from build123d import *

# Parameters (mm, degrees)
F0_W      = 125
F0_H      = 40
F1_DEPTH  = 3
F2_W      = 125
F2_H      = 3
F3_DEPTH  = 85
F4_W      = 125
F4_H      = 40
F5_DEPTH  = 3
F6_R      = 35
F7_DEPTH  = 25
F10_R     = 24
F8_R      = 38
F12_R     = 12.5
F13_DEPTH = 70.6
F16_R     = 18
F14_R     = 35
F18_W     = 70
F18_H     = 3
F19_DEPTH = 85
F20_W     = 60
F20_H     = 60
F21_DEPTH = 15.5
F22_W     = 3
F22_H     = 85
F23_DEPTH = 26
F24_R     = 5
F25_DEPTH = 9.5
F26_R     = 10
F27_DEPTH = 25


with BuildPart() as f1:
    # F0 (on Front) → F1 (new body)
    with BuildSketch(Plane.XZ):
        Rectangle(F0_W, F0_H)
        with BuildLine():
            ThreePointArc((62.5, -20), (82.5, 0), (62.5, 20))
            Line((62.5, 20), (62.5, -20))
        make_face()
        with BuildLine():
            Line((-62.5, -20), (-62.5, 20))
            ThreePointArc((-62.5, 20), (-82.5, 0), (-62.5, -20))
        make_face()
    extrude(amount=F1_DEPTH)

    # F2 (on face) → F3 (join)
    with BuildSketch(Plane.XZ.offset(3)):
        with Locations((0, 18.5)):
            Rectangle(F2_W, F2_H)
        with BuildLine():
            Line((-62.5, 17), (-62.5, 20))
            ThreePointArc((-62.5, 20), (-76.6421356237, 14.1421356237), (-82.5, 0))
            Line((-82.5, 0), (-79.5, 0))
            ThreePointArc((-79.5, 0), (-74.5208152802, 12.0208152802), (-62.5, 17))
        make_face()
        with BuildLine():
            ThreePointArc((82.5, 0), (76.6421356237, 14.1421356237), (62.5, 20))
            Line((62.5, 20), (62.5, 17))
            ThreePointArc((62.5, 17), (74.5208152802, 12.0208152802), (79.5, 0))
            Line((79.5, 0), (82.5, 0))
        make_face()
    extrude(amount=F3_DEPTH)

    # F4 (on face) → F5 (join)
    with BuildSketch(Plane.XZ.offset(88)):
        Rectangle(F4_W, F4_H)
        with BuildLine():
            Line((-62.5, -20), (-62.5, 20))
            ThreePointArc((-62.5, 20), (-82.5, 0), (-62.5, -20))
        make_face()
        with BuildLine():
            ThreePointArc((62.5, -20), (82.5, 0), (62.5, 20))
            Line((62.5, 20), (62.5, -20))
        make_face()
    extrude(amount=F5_DEPTH)

    # F6 (on face) → F7 (cut)
    with BuildSketch(Plane(origin=(0, 0, 17), x_dir=(1, 0, 0), z_dir=(0, 0, -1))):
        with Locations((0, 45.5)):
            Circle(F6_R)
    extrude(amount=-F7_DEPTH, mode=Mode.SUBTRACT)

    # F10 (on offset) → F11 section 0
    with BuildSketch(Plane.XY.offset(64)):
        with Locations((0, -45.5)):
            Circle(F10_R)
    # F8 (on face) → F11 section 1
    with BuildSketch(Plane.XY.offset(20)):
        with Locations((0, -45.5)):
            Circle(F8_R)
    loft()

    # F12 (on face) → F13 (cut)
    with BuildSketch(Plane.XY.offset(64)):
        with Locations((0, -45.5)):
            Circle(F12_R)
    extrude(amount=-F13_DEPTH, mode=Mode.SUBTRACT)

    # F16 (on offset) → F17 section 0
    with BuildSketch(Plane.XY.offset(61)):
        with Locations((0, -45.5)):
            Circle(F16_R)
    # F14 (on face) → F17 section 1
    with BuildSketch(Plane.XY.offset(20)):
        with Locations((0, -45.5)):
            Circle(F14_R)
    loft(mode=Mode.SUBTRACT)

    # F18 (on face) → F19 (join)
    with BuildSketch(Plane.XZ.offset(3)):
        with Locations((0, -4.5)):
            Rectangle(F18_W, F18_H)
    extrude(amount=F19_DEPTH)

    # F20 (on face) → F21 (cut)
    with BuildSketch(Plane(origin=(0, 0, -6), x_dir=(1, 0, 0), z_dir=(0, 0, -1))):
        with Locations((0, 45.5)):
            Rectangle(F20_W, F20_H)
    extrude(amount=-F21_DEPTH, mode=Mode.SUBTRACT)

    # F22 (on face) → F23 (join)
    with BuildSketch(Plane(origin=(0, 0, -6), x_dir=(1, 0, 0), z_dir=(0, 0, -1))):
        with Locations((-33.5, 45.5)):
            Rectangle(F22_W, F22_H)
        with Locations((33.5, 45.5)):
            Rectangle(F22_W, F22_H)
    extrude(amount=-F23_DEPTH)

    # F24 (on face) → F25 (join)
    with BuildSketch(Plane.XZ.offset(3)):
        with Locations((-62.5, 0)):
            Circle(F24_R)
        with Locations((62.5, 0)):
            Circle(F24_R)
    extrude(amount=F25_DEPTH)

    # F26 (on face) → F27 (cut)
    with BuildSketch(Plane.XZ.offset(91)):
        with Locations((-62.5, 0)):
            Circle(F26_R)
        with Locations((62.5, 0)):
            Circle(F26_R)
    extrude(amount=-F27_DEPTH, mode=Mode.SUBTRACT)


solid = f1.part
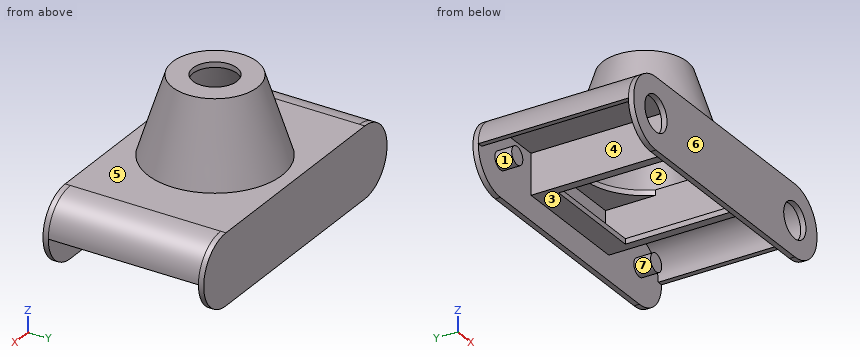
Source: CAD feature listing. Evaluate the final solid. Frame: model axes, mm. Face numbers are marked on the shaded views. A direction names the side the tool comes from. Round coordinates to 2 decimals unless told otherwise and drop trailing zeros. Order: outer loops, then holes, each group sorted by start corner. A loop starts at its lowest first (then second) coordinate and runs counter-clockwise, first axis right, second up. Notation, with made-up numbers: (21.25, 37.25) - (26.25, 37.25) arc R25 cw to (26.25, 49.25) - close; hole circle Ø2 at (27, 45.5). An arc over 180 degrees is marked (long way). Use a Markdown table: item, result. Add a question column.
1. Line query: probe 1 along X at (y, z) = (-58.5, 1); probe 2 along Z at (x, y) = (62.5, -89.1); probe 3 along X at (y, z) = (-23.5, -1.5). Output: solid intervals per line, ascending.
2. Section query C-C (z = 49). Return the cut outline in (x, y), then the cut area to 3 significant figures.
3. Mould query, pull axis Z, two halves, no side actions, for the marked faces 5, 6 and 7. Classes: +Z half, -Z half, draft (parallel to the pull), parting line (faces both ways), or undercut.
4. First-contact query: pin 1 (10 mm diameter, centred on y = -43.5, z = 37.5, fed in from +X); pin 2 (1 mm diameter, centred on y = -81.5, z = 9.5, fed in from +X); pin 3 (14 mm diameter, centred on x = -43, y = -36, fed in from -Z). Flat tips, straight axial feed; report the tip coordinate or a pass-through.
5. Section query B-B (x = 46.5). Return the cut outline in (y, z).
6. Set-up query: the marked faces 1, 2, 3 and 4. Return all of +Z, -Z, +X, -X, +Y, -Y with unobstructed straight access to the full face (end or side cutting, diameter ignored); none if empty.
Derived:
| question | item | result |
|---|---|---|
| 1 | probe 1 | -82.47 to -79.47, -35 to -32, 32 to 35, 79.47 to 82.47 |
| 1 | probe 2 | -20 to -10, 10 to 20 |
| 1 | probe 3 | -35 to -32, 32 to 35 |
| 2 | outline | circle Ø57.55 at (0, -45.5); hole circle Ø45.95 at (0, -45.5) |
| 2 | area | 942 mm2 |
| 3 | face 5 | +Z half |
| 3 | face 6 | draft |
| 3 | face 7 | undercut |
| 4 | pin 1 | x = 33.98 |
| 4 | pin 2 | x = 80.36 |
| 4 | pin 3 | z = 17 |
| 5 | outline | (-91, -20) - (-88, -20) - (-88, 17) - (-3, 17) - (-3, -20) - (0, -20) - (0, 20) - (-91, 20) - close |
| 6 | face 1 | -Y |
| 6 | face 2 | none |
| 6 | face 3 | -Z, +X, -X |
| 6 | face 4 | -Z |
